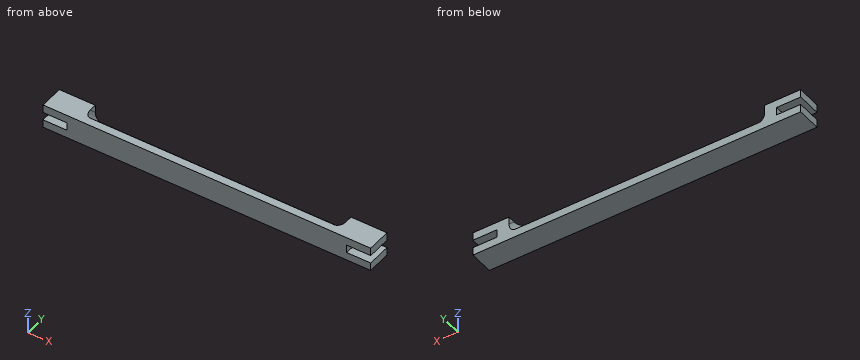
from build123d import *

# Parameters (mm, degrees)
F1_DEPTH = 38.1
F4_DEPTH = 203.2
F5_R     = 9.525


with BuildPart() as f1:
    # F0 (on Front) → F1 (new body)
    with BuildSketch(Plane.XZ):
        Polygon((520.7, 0), (0, 0), (0, -12.7), (38.1, -12.7), (38.1, -25.4), (0, -25.4), (0, -38.1), (520.7, -38.1), (520.7, -25.4), (482.6, -25.4), (482.6, -12.7), (520.7, -12.7), align=None)
    extrude(amount=F1_DEPTH)

    # F3 (on offset) → F4 (cut, symmetric)
    with BuildSketch(Plane.YZ.offset(260.35)):
        Polygon((0, -25.4), (0, 0), (-25.4, 0), align=None)
    extrude(amount=F4_DEPTH, both=True, mode=Mode.SUBTRACT)

    # F5
    f5_edges = [f1.edges().sort_by_distance(p)[0] for p in [
        (463.55, -12.7, -12.7),
        (57.15, -12.7, -12.7),
    ]]
    fillet(f5_edges, radius=F5_R)


solid = f1.part
Here's how the part is built. I have some questions about the finished solid (model axes, mm). Coordinates: 2 decimals unless noted, no trailing zeros. Order: outer loops, then holes, each group sorted by start corner. A loop starts at its lowest first (then second) coordinate and runs counter-clockwise, first axis right, second up. Notation, with made-up numbers: M 47,10 L 61,10 A17 ccw 61,14 Z; hole C 43.5,52.25 d1. An arc over 180 degrees is marked long. Answer as CSV lines item,"result". Start each with the question number.
1. For pin 1 (3 mm diameter, centred on y = -6.5, z = -22, fed in from +X); pin 2 (8 mm diameter, centred on y = -7, z = -17.5, fed in from -X), each with a flat end and sliding along its axis, tell me the tip position at first contact or that it passes through.
2. I want a section at A-A, the plane x = 445.5. Write out the boundary of the cut face in (y, z), and give its area (3 significant figures).
3. I need wall thicknesses on line 1 (Z direction, x = 28.5, y = -11); line 2 (X direction, y = -14.5, z = -19); line 3 (X direction, y = -9, z = -15.5). Which ranges of each line are inside material? Lowest first, please. Write a range as [from, to].
Recorded:
1,pin 1,"stops at x = 482.6"
1,pin 2,"stops at x = 38.1"
2,outline,"M -38.1,-38.1 L 0,-38.1 L 0,-25.4 L -25.4,0 L -38.1,0 Z"
2,area,"1,130 mm2"
3,line 1,"z = [-38.1, -25.4], [-12.7, 0]"
3,line 2,"x = [38.1, 482.6]"
3,line 3,"x = [38.1, 63.25], [457.45, 482.6]"
